```python
from build123d import *

# Parameters (mm, degrees)
F0_W      = 75.6297543388
F0_H      = 25.4
F0_W_2    = 254
F0_H_2    = 12.7
F1_DEPTH  = 254
F3_DEPTH  = 12.7
F4_R      = 101.6
F5_DEPTH  = 76.2
F6_W      = 76.2
F6_H      = 177.8
F7_DEPTH  = 25.4
F8_W      = 127
F8_H      = 177.8
F9_DEPTH  = 25.4
F10_W     = 76.2
F10_H     = 177.8
F11_DEPTH = 25.4
F12_W     = 76.2
F12_H     = 177.8
F13_DEPTH = 25.4
F14_W     = 76.2
F14_H     = 191.3614441931
F15_DEPTH = 25.4
F17_DEPTH = 241.3
F18_W     = 25.4
F18_H     = 25.4
F19_DEPTH = 62.23
F20_DEPTH = 25.4
F21_W     = 25.4
F21_H     = 25.4
F22_DEPTH = 25.4
F23_W     = 77.4427120167
F23_H     = 102.6062965393
F24_DEPTH = 71.12
F25_W     = 39.3790647912
F25_H     = 60.6827586889
F26_DEPTH = 53.34
F27_W     = 32.5816385448
F27_H     = 54.1992932558
F28_DEPTH = 20.32
F29_R     = 2.3092601705
F30_DEPTH = 11.684


with BuildPart() as f1:
    # F0 (on Top) → F1 (new body)
    with BuildSketch(Plane.XY):
        Polygon((-705.2555303436, -766.5243874192), (-578.2555303436, -766.5243874192), (31.3444696564, -766.5243874192), (31.3444696564, -753.8243874192), (31.3444696564, -639.5243874192), (31.3444696564, -182.3243874192), (31.3444696564, -169.6243874192), (31.3444696564, 84.3756125808), (31.3444696564, 97.0756125808), (31.3444696564, 439.9756125808), (31.3444696564, 452.6756125808), (31.3444696564, 554.2756125808), (-578.2555303436, 554.2756125808), (-705.2555303436, 554.2756125808), (-705.2555303436, -639.5243874192), align=None)
        Polygon((-692.5555303436, 236.7756125808), (-692.5555303436, 541.5756125808), (18.6444696564, 541.5756125808), (18.6444696564, -753.8243874192), (-692.5555303436, -753.8243874192), (-692.5555303436, 211.3756125808), align=None, mode=Mode.SUBTRACT)
        Polygon((31.3444696564, -753.8243874192), (31.3444696564, -766.5243874192), (298.0444696564, -766.5243874192), (298.0444696564, 452.6756125808), (31.3444696564, 452.6756125808), (31.3444696564, 439.9756125808), (285.3444696564, 439.9756125808), (285.3444696564, 97.0756125808), (285.3444696564, 84.3756125808), (285.3444696564, -169.6243874192), (285.3444696564, -182.3243874192), (285.3444696564, -753.8243874192), align=None)
        with Locations((-654.7406531742, 224.0756125808)):
            Rectangle(F0_W, F0_H)
        with Locations((158.3444696564, -175.9743874192)):
            Rectangle(F0_W_2, F0_H_2)
        with Locations((158.3444696564, 90.7256125808)):
            Rectangle(F0_W_2, F0_H_2)
    extrude(amount=-F1_DEPTH)

    # F2 (on face) → F3 (join)
    with BuildSketch(Plane(origin=(0, 0, -254), x_dir=(1, 0, 0), z_dir=(0, 0, -1))):
        Polygon((-705.2555303436, -554.2756125808), (-692.5555303436, -554.2756125808), (31.3444696564, -554.2756125808), (31.3444696564, -452.6756125808), (298.0444696564, -452.6756125808), (298.0444696564, 766.5243874192), (-705.2555303436, 766.5243874192), align=None)
    extrude(amount=-F3_DEPTH)

    # F4 (on face) → F5 (join)
    with BuildSketch(Plane.XY.offset(-241.3)):
        with Locations((-409.7238771986, -11.7228467155)):
            Circle(F4_R)
        with Locations((-219.1344722543, -194.9250362249)):
            Circle(F4_R)
        with Locations((-439.272572652, -366.3077359129)):
            Circle(F4_R)
        with Locations((-222.0893417996, -524.3934827381)):
            Circle(F4_R)
    extrude(amount=F5_DEPTH)

    # F6 (on face) → F7 (cut)
    with BuildSketch(Plane.YZ.offset(-692.5555303436)):
        with Locations((309.93842659, -152.4)):
            Rectangle(F6_W, F6_H)
    extrude(amount=-F7_DEPTH, mode=Mode.SUBTRACT)

    # F8 (on face) → F9 (cut)
    with BuildSketch(Plane(origin=(0, -753.8243874192, 0), x_dir=(-1, 0, 0), z_dir=(0, 1, 0))):
        with Locations((248.0555303436, -152.4)):
            Rectangle(F8_W, F8_H)
    extrude(amount=-F9_DEPTH, mode=Mode.SUBTRACT)

    # F10 (on face) → F11 (cut)
    with BuildSketch(Plane(origin=(18.6444696564, 0, 0), x_dir=(0, -1, 0), z_dir=(-1, 0, 0))):
        with Locations((233.1243874192, -152.4)):
            Rectangle(F10_W, F10_H)
        with Locations((563.3243874192, -152.4)):
            Rectangle(F10_W, F10_H)
        with Locations((118.8243874192, -152.4)):
            Rectangle(F10_W, F10_H)
    extrude(amount=-F11_DEPTH, mode=Mode.SUBTRACT)

    # F12 (on face) → F13 (cut)
    with BuildSketch(Plane.XZ.offset(-84.3756125808)):
        with Locations((89.0679913521, -152.4)):
            Rectangle(F12_W, F12_H)
    extrude(amount=-F13_DEPTH, mode=Mode.SUBTRACT)

    # F14 (on face) → F15 (cut)
    with BuildSketch(Plane.YZ.offset(31.3444696564)):
        with Locations((490.7756125808, -145.6192779034)):
            Rectangle(F14_W, F14_H)
    extrude(amount=-F15_DEPTH, mode=Mode.SUBTRACT)

    # F16 (on face) → F17 (join)
    with BuildSketch(Plane.XY.offset(-241.3)):
        Polygon((-53.3087753415, 236.7756125808), (-78.7087753415, 236.7756125808), (-78.7087753415, 211.3756125808), (-61.1483082175, 211.3756125808), (-53.3087753415, 211.3756125808), align=None)
    extrude(amount=F17_DEPTH)

    # F18 (on face) → F19 (join)
    with BuildSketch(Plane.XY.offset(-241.3)):
        with Locations((-498.9669535637, 368.9300801277)):
            Rectangle(F18_W, F18_H)
        with Locations((-498.9669535637, 279.9933936119)):
            Rectangle(F18_W, F18_H)
        with Locations((-383.7003324509, 279.9933936119)):
            Rectangle(F18_W, F18_H)
        with Locations((-383.7003324509, 368.9300801277)):
            Rectangle(F18_W, F18_H)
    extrude(amount=F19_DEPTH)

    # F18 (on face) → F20 (join)
    with BuildSketch(Plane.XY.offset(-241.3)):
        with Locations((-498.9669535637, 368.9300801277)):
            Rectangle(F18_W, F18_H)
        with Locations((-498.9669535637, 279.9933936119)):
            Rectangle(F18_W, F18_H)
        with Locations((-383.7003324509, 279.9933936119)):
            Rectangle(F18_W, F18_H)
        with Locations((-383.7003324509, 368.9300801277)):
            Rectangle(F18_W, F18_H)
    extrude(amount=F20_DEPTH)

    # F21 (on face) → F22 (join)
    with BuildSketch(Plane.XY.offset(-179.07)):
        with Locations((-498.9669535637, 368.9300801277)):
            Rectangle(F21_W, F21_H)
        Polygon((-486.2669535637, 356.2300801277), (-511.6669535637, 356.2300801277), (-511.6669535637, 267.2933936119), (-396.4003324509, 267.2933936119), (-396.4003324509, 292.6933936119), (-371.0003324509, 292.6933936119), (-371.0003324509, 381.6300801277), (-486.2669535637, 381.6300801277), align=None)
        with Locations((-383.7003324509, 279.9933936119)):
            Rectangle(F21_W, F21_H)
    extrude(amount=F22_DEPTH)

    # F23 (on face) → F24 (join)
    with BuildSketch(Plane.XY.offset(-241.3)):
        with Locations((-20.076886352, -393.2565152645)):
            Rectangle(F23_W, F23_H)
    extrude(amount=F24_DEPTH)

    # F25 (on face) → F26 (join)
    with BuildSketch(Plane.XY.offset(-241.3)):
        with Locations((-1.0450627392, 133.5669532418)):
            Rectangle(F25_W, F25_H)
    extrude(amount=F26_DEPTH)

    # F27 (on face) → F28 (cut)
    with BuildSketch(Plane.XY.offset(-187.96)):
        with Locations((-1.1091437191, 133.5575208068)):
            Rectangle(F27_W, F27_H)
    extrude(amount=-F28_DEPTH, mode=Mode.SUBTRACT)

    # F29 (on face) → F30 (cut)
    with BuildSketch(Plane.XY.offset(-208.28)):
        with Locations((0, 133.9616626501)):
            Circle(F29_R)
    extrude(amount=-F30_DEPTH, mode=Mode.SUBTRACT)


solid = f1.part
```
CAD build for the part. Positions are in the model's coordinates, mm. A direction names the side the tool comes from. Round coordinates to 2 decimals unless told otherwise and drop trailing zeros. Order: outer loops, then holes, each group sorted by start corner. A loop starts at its lowest first (then second) coordinate and runs counter-clockwise, first axis right, second up. Notation, with made-up numbers: (-17.75, -23) - (11.25, -23) arc R29 cw to (11.25, 1) - close; hole circle Ø2 at (43.5, 2). An arc over 180 degrees is marked (long way). Answer in a Markdown table with one row per item. Add a question column.
(1) Mould opens along X. For faces 5 (the face through (-384, 292.693, -211)), 6 (the face through (-66, 236.776, -122)) say: +X half, -X half, draft (parallel to the pull), parting line (faces both ways), or undercut.
(2) Probe L1, parallel to X at y = 179, z = -34.5; L2, parallel to X at y = 147, z = -195; L3, parallel to Y at x = 153.5, z = -78. List the from-to ranges inside material, lowest first. Write a range as [from, to].
(3) Band-saw the part on C-C on z = -112. Count the separate pieces of the cut face and the enclosed holes in it, and give its area (3 significant figures).
(4) Band-saw the part on B-B on x = -283. List the corners of the cut face in (y, z).
(5) Drop flat-ended pins along their axis: pin 1 Ø4 at (x, y) = (80, -470.5) entering from +Z; pin 2 Ø2.5 at (x, y) = (0, 133.5) entering from +Z; pin 3 Ø1.5 at (x, y) = (-175.5, -270.5) entering from +Z. Give the stop position or say it passes through.
(6) Band-saw the part on D-D on x = 192. List the corners of the cut face in (y, z).
(7) Band-saw the part on A-A on y = -579. List the corners of the cut face in (x, z), and give its area (3 significant figures).
(8) 3-axis set-ups, long thin cutter, end or side, ignore diameter. For faces 1 (the face through (-312.816, 18.795, -203.733)), 2 (the face through (-384, 356.23, -211)), 3 (the face through (-211, -766.524, -41)), 4 (the face through (-499, 292.693, -211)): which of +Z, -Z, +X, -X, +Y, -Y reach the whole face in a straight line?
Data:
| question | item | result |
|---|---|---|
| 1 | face 5 | draft |
| 1 | face 6 | undercut |
| 2 | L1 | x = [-705.26, -692.56], [18.64, 31.34], [285.34, 298.04] |
| 2 | L2 | x = [-705.26, -692.56], [-20.73, -17.4], [15.18, 31.34], [285.34, 298.04] |
| 2 | L3 | y = [-766.52, -753.82], [-182.32, -169.62], [84.38, 97.08], [439.98, 452.68] |
| 3 | separate pieces | 5 |
| 3 | enclosed holes | 0 |
| 3 | area | 75,100 mm^2 |
| 4 | outline | (-766.52, -254) - (554.28, -254) - (554.28, 0) - (541.58, 0) - (541.58, -241.3) - (-115.91, -241.3) - (-115.91, -165.1) - (-273.94, -165.1) - (-273.94, -241.3) - (-443.08, -241.3) - (-443.08, -165.1) - (-605.71, -165.1) - (-605.71, -241.3) - (-766.52, -241.3) - close; (-766.52, -63.5) - (-753.82, -63.5) - (-753.82, 0) - (-766.52, 0) - close |
| 5 | pin 1 | stops at z = -241.3 |
| 5 | pin 2 | stops at z = -219.96 |
| 5 | pin 3 | stops at z = -165.1 |
| 6 | outline | (-766.52, -254) - (452.68, -254) - (452.68, 0) - (439.98, 0) - (439.98, -241.3) - (97.08, -241.3) - (97.08, 0) - (84.38, 0) - (84.38, -241.3) - (-169.62, -241.3) - (-169.62, 0) - (-182.32, 0) - (-182.32, -241.3) - (-753.82, -241.3) - (-753.82, 0) - (-766.52, 0) - close |
| 7 | outline | (-705.26, -254) - (298.04, -254) - (298.04, 0) - (285.34, 0) - (285.34, -241.3) - (-136.41, -241.3) - (-136.41, -165.1) - (-307.77, -165.1) - (-307.77, -241.3) - (-692.56, -241.3) - (-692.56, 0) - (-705.26, 0) - close; (18.64, -63.5) - (31.34, -63.5) - (31.34, 0) - (18.64, 0) - close |
| 7 | area | 32,700 mm^2 |
| 8 | face 1 | +Z |
| 8 | face 2 | none |
| 8 | face 3 | +Z, -Z, +X, -X, -Y |
| 8 | face 4 | -X |
